```python
from build123d import *

# Parameters (mm, degrees)
SKETCH1_R           = 4
SKETCH1_R_2         = 2.5
SKETCH1_R_3         = 6.5
BOSS_EXTRUDE1_DEPTH = 6.2
CUT_EXTRUDE1_REACH  = 278.492
SKETCH2_R           = 1.5


with BuildPart() as part:
    # Sketch1 → Boss-Extrude1 (new body)
    with BuildSketch(Plane.XY):
        with BuildLine():
            ThreePointArc((-4.843381354, 29.606446208), (-29.489039073, -5.513308858), (6.180402599, -29.356474988))
            ThreePointArc((6.180402599, -29.356474988), (128.63005147, -16.382678773), (251.170355628, -28.47026553))
            ThreePointArc((251.170355628, -28.47026553), (273.303133895, -14.765534175), (260.982883768, 8.166778664))
            ThreePointArc((260.982883768, 8.166778664), (129.376669821, 35.090841966), (-4.843381354, 29.606446208))
        make_face()
        with Locations(Location((254.95, -9.85, 0), (0, 0, 180))):
            Circle(SKETCH1_R, mode=Mode.SUBTRACT)
        with Locations(Location((0, 23, 0), (0, 0, 180))):
            Circle(SKETCH1_R_2, mode=Mode.SUBTRACT)
        with Locations(Location((0, -23, 0), (0, 0, 180))):
            Circle(SKETCH1_R_2, mode=Mode.SUBTRACT)
        with Locations(Location((-23, 0, 0), (0, 0, 180))):
            Circle(SKETCH1_R_2, mode=Mode.SUBTRACT)
        with Locations(Location((23, 0, 0), (0, 0, 180))):
            Circle(SKETCH1_R_2, mode=Mode.SUBTRACT)
        with Locations(Location((0, 0, 0), (0, 0, 180))):
            Circle(SKETCH1_R_3, mode=Mode.SUBTRACT)
        with BuildLine():
            Line((85.299988347, 14.334161591), (86.047515876, 3.894174942))
            ThreePointArc((86.047515876, 3.894174942), (88.416575223, -0.870831987), (93.451584576, -2.593160073))
            ThreePointArc((93.451584576, -2.593160073), (129.051714651, -1.468455886), (164.657677356, -2.390215498))
            ThreePointArc((164.657677356, -2.390215498), (169.415573807, -0.864394835), (171.943987902, 3.445225739))
            Line((171.943987902, 3.445225739), (172.629734019, 7.547504331))
            ThreePointArc((172.629734019, 7.547504331), (171.396804828, 12.804877005), (166.788880257, 15.62038992))
            ThreePointArc((166.788880257, 15.62038992), (129.692411097, 20.014503602), (92.380913243, 21.833400801))
            ThreePointArc((92.380913243, 21.833400801), (87.192448356, 19.639856576), (85.299988347, 14.334161591))
        make_face(mode=Mode.SUBTRACT)
    extrude(amount=BOSS_EXTRUDE1_DEPTH)

    # Sketch2 → Cut-Extrude1 (cut, up to next)
    with BuildSketch(Plane.XY.offset(6.2), mode=Mode.PRIVATE) as cut_extrude1_sk1:
        with Locations((-4.75, -8.227241336)):
            Circle(SKETCH2_R)
    cut_extrude1_tool1 = extrude(cut_extrude1_sk1.sketch, amount=-CUT_EXTRUDE1_REACH, mode=Mode.PRIVATE) & part.part
    # Sketch2 → Cut-Extrude1 (cut, up to next)
    with BuildSketch(Plane.XY.offset(6.2), mode=Mode.PRIVATE) as cut_extrude1_sk2:
        with Locations((-4.75, 8.227241336)):
            Circle(SKETCH2_R)
    cut_extrude1_tool2 = extrude(cut_extrude1_sk2.sketch, amount=-CUT_EXTRUDE1_REACH, mode=Mode.PRIVATE) & part.part
    # Sketch2 → Cut-Extrude1 (cut, up to next)
    with BuildSketch(Plane.XY.offset(6.2), mode=Mode.PRIVATE) as cut_extrude1_sk3:
        with Locations((9.5, 0)):
            Circle(SKETCH2_R)
    cut_extrude1_tool3 = extrude(cut_extrude1_sk3.sketch, amount=-CUT_EXTRUDE1_REACH, mode=Mode.PRIVATE) & part.part
    add(cut_extrude1_tool1.solids().sort_by_distance((-4.75, -8.227241, 6.2))[0], mode=Mode.SUBTRACT)
    add(cut_extrude1_tool2.solids().sort_by_distance((-4.75, 8.227241, 6.2))[0], mode=Mode.SUBTRACT)
    add(cut_extrude1_tool3.solids().sort_by_distance((9.5, 0, 6.2))[0], mode=Mode.SUBTRACT)


solid = part.part
```
Input: part model. Units: mm. Frame: model coordinates. A direction names the side the tool comes from. Coordinates: 2 decimals unless noted, no trailing zeros. Write each loop counter-clockwise with the first axis right and the second up, starting at its lowest first coordinate (ties: lowest second). Pieces come first, ordered by that corner, then holes. Notation, with made-up numbers: M 37,45.5 L 72,45.5 A34 cw 72,83.5 Z; hole C 67,50 d8. An arc over 180 degrees is marked long. Use one line per item in the form item = value.
Q1. Section A-A (x = 254.95). Return loops of the section in (y, z), plus the area to 3 significant figures.
Answer below:
outline = M -28.85,0 L -13.85,0 L -13.85,6.2 L -28.85,6.2 Z; M -5.85,0 L 10.15,0 L 10.15,6.2 L -5.85,6.2 Z
area = 192 mm²
Q2. Section D-D (x = 82). Return loops of the section in (y, z).
Answer below:
outline = M -18.35,0 L 36.88,0 L 36.88,6.2 L -18.35,6.2 Z
Q3. Set-up query: faces 1 (the face through (171.442, 12.742, 3.057)), 2 (the face through (120, -4, 6.2)). Return all of +Z, -Z, +X, -X, +Y, -Y with unobstructed straight access to the full face (end or side cutting, diameter ignored); none if empty.
Answer below:
face_1 = +Z, -Z
face_2 = +Z, +X, -X, +Y, -Y
Q4. Material intervals for probe 1 along Y at (x, z) = (-4.75, 4.75); probe 2 along X at (y, z) = (5.5, 5.25); probe 3 along Y at (x, z) = (23, 2), sorted ascending. Write a range as from..to.
Answer below:
probe_1 = -29.62..-9.73, -6.73..-4.44, 4.44..6.73, 9.73..29.62
probe_2 = -29.49..-3.46, 3.46..85.93, 172.29..266.15
probe_3 = -26.06..-2.5, 2.5..33.44
Q5. First-contact query: pin 1 (2.5 mm diameter, centred on x = -4.75, y = 8.23, fed in from -Z); pin 2 (1 mm diameter, centred on y = -22.5, z = 3.5, fed in from +X); pin 3 (1.5 mm diameter, centred on y = -18.5, z = 4.5, fed in from -X). Flat tips, straight axial feed; report the tip coordinate or a pass-through.
Answer below:
pin_1 = through
pin_2 = 269.56
pin_3 = -24.19
Q6. Section B-B (z = 4.25). Count the separate pieces of the cut face and the enclosed holes in it, plus the area to 3 significant figures.
Answer below:
separate_pieces = 1
enclosed_holes = 10
area = 12,900 mm²
Q7. Section C-C (x = -23). Return loops of the section in (y, z).
Answer below:
outline = M -19.26,0 L -2.5,0 L -2.5,6.2 L -19.26,6.2 Z; M 2.5,0 L 19.26,0 L 19.26,6.2 L 2.5,6.2 Z
Q8. Draft query along X for faces 3 (the face through (120, -4, 0)), 4 (the face through (88.36, -0.82, 3.06)), 5 (the face through (131.256, 34.936, 3.057)). Return one class per face: released by +X, released by -X, zero draft, split by the parting line, or undercut.
Answer below:
face_3 = zero draft
face_4 = undercut
face_5 = split by the parting line
